Source: three-view drawing plus pictorial views. Frame: mm from the lowest corner of the part. A direction names the side the tool comes from. Coordinates: 2 decimals unless noted, no trailing zeros. Order: outer loops, then holes, each group sorted by start corner. A loop starts at its lowest first (then second) coordinate and runs counter-clockwise, first axis right, second up. Notation, with made-up numbers: (46, 12.25) -> (59, 12.25) arc R31 ccw to (59, 41.25) -> close; hole circle Ø1 at (3, 12.5). An arc over 180 degrees is marked (long way). Use one line per item in the form item = value. Start each with the question number.
1) Section query B-B on z = 5.5. Count the separate pieces of the cut face and the enclosed holes in it, then the cut area to 3 significant figures.
2) Section query A-A on x = 8.25. Output: boundary loops of the cut face in (y, z).
3) Access query for the marked faces 1, 2, 3, 4 and 5. Directions: +Z, -Z, +X, -X, +Y, -Y. A direction counts if a zero-diameter tool reaches every point of the face in a straight line with its end or side. Return the directions, or none.
4) Draft query along X for the marked faces 6, 7 and 8. Return one class per face: pulls with the +X half, pulls with the -X half, needs draft (parallel to the pull), parting line crosses it, or undercut.
5) Pin query (flat end, axial travel): pin 1 (3 mm diameter, centred on x = 8.5, z = 7.5, fed in from +Y); pin 2 (5 mm diameter, centred on x = 4, z = 6, fed in from -Y); pin 3 (5.5 mm diameter, centred on y = 4, z = 4.5, fed in from -X). Return the tip coordinate at first contact, or that it passes through.
6) Ray query, line 1 along Z through (x, y) = (16.5, 39.5); line 2 along Y through (x, z) = (5.5, 2); line 3 along Y through (x, z) = (16.75, 5.5) (1 decimal). Return the intervals inside material, ascending.
7) Section query D-D on y = 30.5. Output: boundary loops of the cut face in (x, z), then the cut area to 3 significant figures.
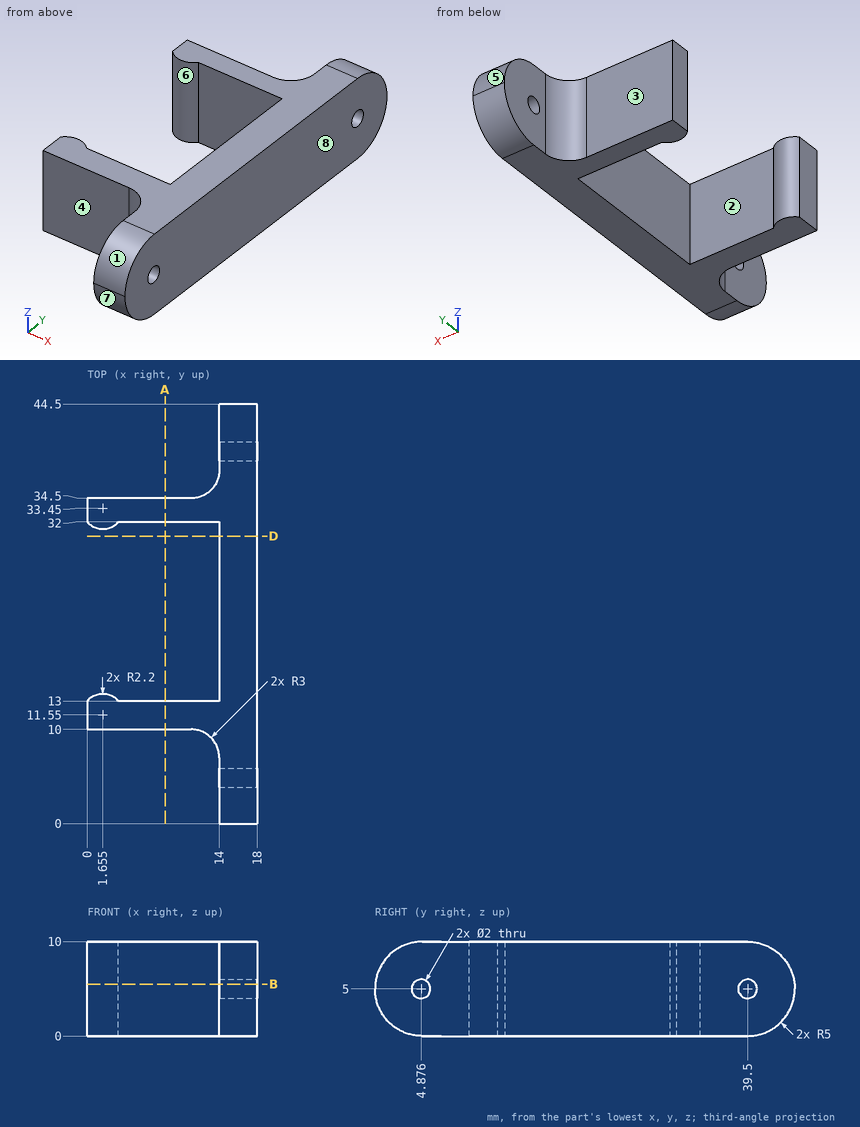
Answers below:
q1.separate_pieces = 3
q1.enclosed_holes = 0
q1.area = 248 mm^2
q2.outline = (10, 0) -> (13, 0) -> (13, 10) -> (10, 10) -> close; (32, 0) -> (34.5, 0) -> (34.5, 10) -> (32, 10) -> close
q3.face_1 = +Z, +X, -X, -Y
q3.face_2 = +Z, -Z
q3.face_3 = +Z, -Z, -X, +Y
q3.face_4 = +Z, -Z, -X, -Y
q3.face_5 = +Z, +X, -X, +Y
q4.face_6 = undercut
q4.face_7 = needs draft
q4.face_8 = pulls with the +X half
q5.pin_1 = 34.5
q5.pin_2 = 10
q5.pin_3 = 14
q6.line_1 = 0 to 4, 6 to 10
q6.line_2 = 10 to 13, 32 to 34.5
q6.line_3 = 0 to 4, 5.7 to 38.6, 40.4 to 44.5
q7.outline = (14, 0) -> (18, 0) -> (18, 10) -> (14, 10) -> close
q7.area = 40.0 mm^2
